The model under review builds one solid part; all positions refer to its coordinate system, in mm. A direction names the side the tool comes from. Round coordinates to 2 decimals unless told otherwise and drop trailing zeros. Order: outer loops, then holes, each group sorted by start corner. A loop starts at its lowest first (then second) coordinate and runs counter-clockwise, first axis right, second up. Notation, with made-up numbers: M 20.5,-36.75 L 36.5,-36.75 A16 ccw 36.5,-18.75 Z; hole C 11.5,36.5 d2. An arc over 180 degrees is marked long. Answer as a JSON object with one key per item and string values. Group by question number.
1) The part is to be moulded in two halves that separate along X. For faces 1 (the flat face through (-2, 0, -1)), 2 (the cylindrical face through (97.619, 24.65, -5.585)), 3 (the cylindrical face through (-88.381, 4.93, -5.585)), 4 (the flat face through (113.5, 25, 1)), say which applies: +X half, -X half, draft (parallel to the pull), parting line (faces both ways), or undercut.
2) Insertion check: pin 1 Ø3 at (y, z) = (23, 10) entering from -X; pin 2 Ø21 at (x, z) = (-102.5, -17) entering from +Y. Each pin has a flat end and moves straight along its axis. Give the tip position at first contact, or say it passes through.
3) For faces 5 (the flat face through (-2, 25, -40)), 6 (the flat face through (-72, 30, -7)), list the 3-axis set-ups (+Z, -Z, +X, -X, +Y, -Y) from which the entire face can be reached by the end or side of a thin tool; tool diameter is ignored.
4) Consider section A-A, the plane x = -93. Write out the cut boundary in (y, z).
5) To check wall thickness, follow line 1 (X direction, y = 3.5, z = -7.5); line 2 (X direction, y = 11, z = -7); line 3 (Z direction, x = 93, y = 27.5). State the ranges of each line that lie inside material, in increasing order.
6) Consider section B-B, the plane y = 28.5. Write out the cut boundary in (x, z), then the cut area to 3 significant figures.
7) Consider section D-D, the plane x = 93. Write out the cut boundary in (y, z), then the cut area to 3 significant figures.
8) Consider section C-C, the plane z = -7.5. Write out the cut boundary in (x, y).
```python
from build123d import *

# Parameters (mm, degrees)
SKETCH1_W           = 227
SKETCH1_H           = 80
SKETCH1_R           = 5
BOSS_EXTRUDE1_DEPTH = 50
SKETCH2_W           = 42
SKETCH2_H           = 42
CUT_EXTRUDE1_DEPTH  = 40


with BuildPart() as part:
    # Sketch1 → Boss-Extrude1 (new body)
    with BuildSketch(Plane(origin=(0, 0, 0), x_dir=(1, 0, 0), z_dir=(0, 1, 0))):
        Rectangle(SKETCH1_W, SKETCH1_H)
        with Locations((-93, 7.5)):
            Circle(SKETCH1_R, mode=Mode.SUBTRACT)
        with Locations((93, 7.5)):
            Circle(SKETCH1_R, mode=Mode.SUBTRACT)
    extrude(amount=BOSS_EXTRUDE1_DEPTH)

    # Sketch2 → Cut-Extrude1 (cut)
    with BuildSketch(Plane(origin=(0, 50, 0), x_dir=(1, 0, 0), z_dir=(0, 1, 0))):
        with Locations((-93, 7.5)):
            Rectangle(SKETCH2_W, SKETCH2_H)
    extrude(amount=-CUT_EXTRUDE1_DEPTH, mode=Mode.SUBTRACT)


solid = part.part
```
Results list:
{
 "1": {"face 1": "draft", "face 2": "undercut", "face 3": "undercut", "face 4": "+X half"},
 "2": {"pin 1": "x = -72", "pin 2": "y = 10"},
 "3": {"face 5": "-Z, +X, -X, +Y, -Y", "face 6": "-X, +Y"},
 "4": {"outline": "M 0,-40 L 50,-40 L 50,-28.5 L 10,-28.5 L 10,-12.5 L 0,-12.5 Z; M 0,-2.5 L 10,-2.5 L 10,13.5 L 50,13.5 L 50,40 L 0,40 Z"},
 "5": {"line 1": "-113.5 to -98, -88 to 88, 98 to 113.5", "line 2": "-72 to 88.03, 97.97 to 113.5", "line 3": "-40 to -12.5, -2.5 to 40"},
 "6": {"outline": "M -113.5,-40 L 113.5,-40 L 113.5,40 L -113.5,40 L -113.5,13.5 L -72,13.5 L -72,-28.5 L -113.5,-28.5 Z; hole C 93,-7.5 d10", "area": "16,300 mm^2"},
 "7": {"outline": "M 0,-40 L 50,-40 L 50,-12.5 L 0,-12.5 Z; M 0,-2.5 L 50,-2.5 L 50,40 L 0,40 Z", "area": "3,500 mm^2"},
 "8": {"outline": "M -113.5,0 L -98,0 L -98,10 L -113.5,10 Z; M -88,0 L 88,0 L 88,50 L -72,50 L -72,10 L -88,10 Z; M 98,0 L 113.5,0 L 113.5,50 L 98,50 Z"}
}
